CAD build for the part. Positions are in the model's coordinates, mm. Face numbers are marked on the shaded views. Round coordinates to 2 decimals unless told otherwise and drop trailing zeros. Answer in a Markdown table with one row per item. Add a question column.
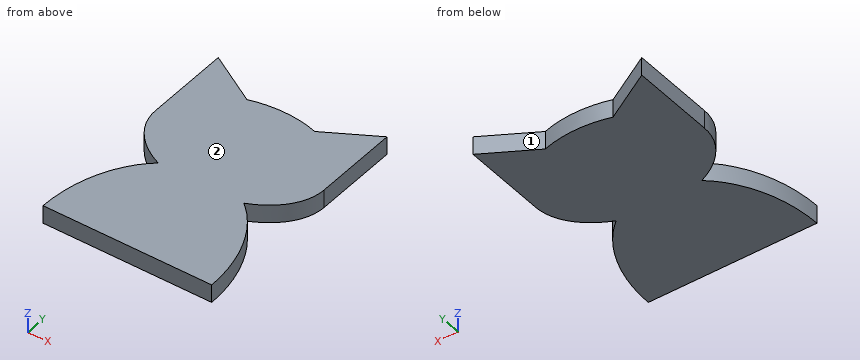
```python
from build123d import *

# Parameters (mm, degrees)
SALIENTE_EXTRUIR2_DEPTH = 3


with BuildPart() as part:
    # Croquis1 → Saliente-Extruir2 (new body)
    with BuildSketch(Plane.XY):
        with BuildLine():
            Line((11, 25), (11, 39))
            Line((11, 39), (19.383258886, 34.159923226))
            add(Edge.make_bspline(
                [(30.616741114, 34.159923226), (25, 35.917122069), (19.383258886, 34.159923226)],
                knots=[4.299567044, 4.299567044, 4.299567044, 5.125210917, 5.125210917, 5.125210917], degree=2, weights=[1, 0.915992323, 1]))
            Line((30.616741114, 34.159923226), (39, 39))
            Line((39, 39), (39, 25))
            add(Edge.make_bspline(
                [(32.095073738, 16.379310345), (39, 19.278775383), (39, 25)],
                knots=[2.102254565, 2.102254565, 2.102254565, 3.141592654, 3.141592654, 3.141592654], degree=2, weights=[1, 0.867983577, 1]))
            add(Edge.make_bspline(
                [(39, 0), (39, 10.870326773), (32.095073738, 16.379310345)],
                knots=[4.71238898, 4.71238898, 4.71238898, 5.751727069, 5.751727069, 5.751727069], degree=2, weights=[1, 0.867983577, 1]))
            Line((39, 0), (11, 0))
            add(Edge.make_bspline(
                [(17.904926262, 16.379310345), (11, 10.870326773), (11, 0)],
                knots=[0.531458238, 0.531458238, 0.531458238, 1.570796327, 1.570796327, 1.570796327], degree=2, weights=[1, 0.867983577, 1]))
            add(Edge.make_bspline(
                [(11, 25), (11, 19.278775383), (17.904926262, 16.379310345)],
                knots=[0, 0, 0, 1.039338089, 1.039338089, 1.039338089], degree=2, weights=[1, 0.867983577, 1]))
        make_face()
    extrude(amount=SALIENTE_EXTRUIR2_DEPTH)


solid = part.part
```
Item 1: Two-plate mould, pull along X, no slides. Class the marked faces 1 and 2: +X half, -X half, draft (parallel to the pull), parting line (faces both ways), or undercut.
Item 2: Drill centre lines: probe 1 along Y at (x, z) = (14.5, 2.15); probe 2 along Y at (x, z) = (34.75, 1.6); probe 3 along X at (y, z) = (20, 2.35). Where is each one in solid material? Low to high.
Item 3: Pin check, flat tip, straight feed: pin 1 (4 mm diameter, centred on x = 22, y = 8, fed in from -Z). Stop position of the tip, or through.
Recorded:
| question | item | result |
|---|---|---|
| 1 | face 1 | undercut |
| 1 | face 2 | draft |
| 2 | probe 1 | 0 to 12.57, 18.39 to 36.98 |
| 2 | probe 2 | 0 to 13.63, 17.82 to 36.55 |
| 2 | probe 3 | 12.88 to 37.12 |
| 3 | pin 1 | z = 0 |
